Source: three-view drawing plus pictorial views. Frame: mm from the lowest corner of the part. A direction names the side the tool comes from. Coordinates: 2 decimals unless noted, no trailing zeros. Write each loop counter-clockwise with the first axis right and the second up, starting at its lowest first coordinate (ties: lowest second). Pieces come first, ordered by that corner, then holes. Notation, with made-up numbers: (-9.5, 48.5) -> (11.5, 48.5) arc R10 ccw to (11.5, 65.5) -> close; hole circle Ø6 at (-21.5, -28). An arc over 180 degrees is marked (long way). Write item = value, one per line.
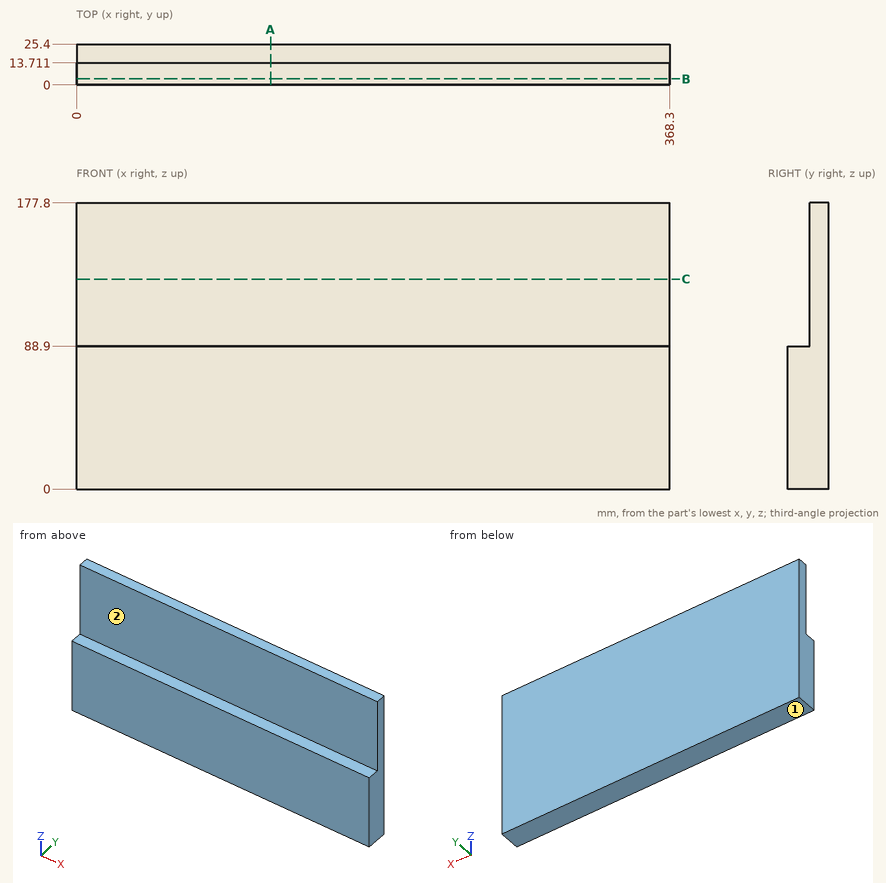
1) Material intervals for probe 1 along Z at (x, y) = (222, 1.75); probe 2 along Y at (x, z) = (171, 92), sorted ascending. Write a range as [from, to].
Answer block:
probe_1 = [0, 88.9]
probe_2 = [13.71, 25.4]
2) Cut plane B-B, the plane y = 3.75. Output: boundary loops of the cut face in (x, z), and give its area (3 significant figures).
Answer block:
outline = (0, 0) -> (368.3, 0) -> (368.3, 88.9) -> (0, 88.9) -> close
area = 32,700 mm2
3) Cut plane A-A, the plane x = 120.5. Output: boundary loops of the cut face in (y, z), and give its area (3 significant figures).
Answer block:
outline = (0, 0) -> (25.4, 0) -> (25.4, 177.8) -> (13.71, 177.8) -> (13.71, 88.9) -> (0, 88.9) -> close
area = 3,300 mm2
4) Cut plane C-C, the plane z = 130.5. Output: boundary loops of the cut face in (x, y).
Answer block:
outline = (0, 13.71) -> (368.3, 13.71) -> (368.3, 25.4) -> (0, 25.4) -> close
5) First-contact query: pin 1 Ø4 at (x, y) = (246, 5) entering from +Z. Flat tip, straight axial feed; report the tip coordinate or a pass-through.
Answer block:
pin_1 = 88.9
6) Reachability of the marked faces 1 and 2 from +Z, -Z, +X, -X, +Y, -Y: full face, straight path, thin tool, end or side. Return the list, or none.
Answer block:
face_1 = -Z, +X, -X, +Y, -Y
face_2 = +Z, +X, -X, -Y
